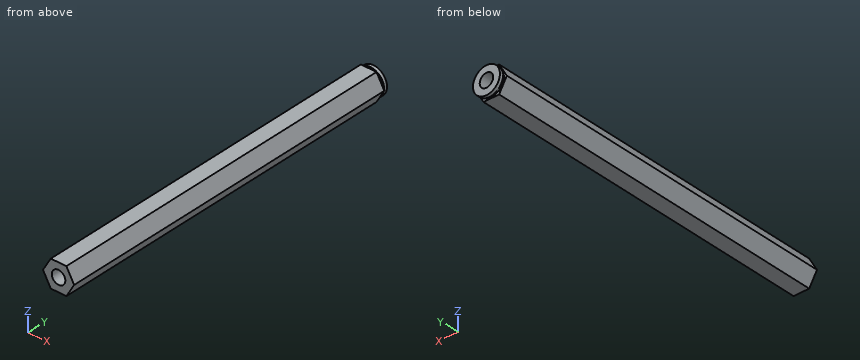
```python
from build123d import *

# Parameters (mm, degrees)
F0_R     = 3.175
F1_DEPTH = 168.275


with BuildPart() as f1:
    # F0 (on Front) → F1 (new body)
    with BuildSketch(Plane.XZ):
        Polygon((3.6661742094, 6.35), (-3.6661742094, 6.35), (-7.3323484187, 0), (-3.6661742094, -6.35), (3.6661742094, -6.35), (7.3323484187, 0), align=None)
        Circle(F0_R, mode=Mode.SUBTRACT)
    extrude(amount=F1_DEPTH)

    # F2 (on Top) → F3 (revolve, cut)
    with BuildSketch(Plane.XY):
        Polygon((-6.35, -1.5875), (-6.35, 0), (-7.3323484187, 0), (-7.3323484187, -2.5781), (-5.9436, -2.5781), (-5.9436, -1.5875), align=None)
    revolve(axis=Axis((0, -1.28905, 0), (0, -1, 0)), mode=Mode.SUBTRACT)


solid = f1.part
```
Input: part model. Units: mm. Frame: model coordinates. Give positions to 0.01 mm unless a question says otherwise; leave off trailing zeros. Order: outer loops, then holes, each group sorted by start corner. A loop starts at its lowest first (then second) coordinate and runs counter-clockwise, first axis right, second up.
1. Section C-C on z = 1.5. Return the cut outline in (x, y) (1 decimal).
Derived:
outline: (-6.5, -168.3) - (-2.8, -168.3) - (-2.8, 0) - (-6.2, 0) - (-6.2, -1.6) - (-5.8, -1.6) - (-5.8, -2.6) - (-6.5, -2.6) - close; (2.8, -168.3) - (6.5, -168.3) - (6.5, -2.6) - (5.8, -2.6) - (5.8, -1.6) - (6.2, -1.6) - (6.2, 0) - (2.8, 0) - close
2. Section B-B on y = -94. Return the cut outline in (x, z) (3 decimals).
Derived:
outline: (-7.332, 0) - (-3.666, -6.35) - (3.666, -6.35) - (7.332, 0) - (3.666, 6.35) - (-3.666, 6.35) - close; hole circle Ø6.35 at (0, 0)
3. Material intervals for L1, parallel to Z at x = 0, y = -75.5 (3 decimals); L2, parallel to X at y = -7, z = 1 (3 decimals); L3, parallel to X at y = -21.5, z = -1.5, sorted ascending.
Derived:
L1: z = -6.35 to -3.175, 3.175 to 6.35
L2: x = -6.755 to -3.013, 3.013 to 6.755
L3: x = -6.47 to -2.8, 2.8 to 6.47
4. Pin query (flat end, axial travel): pin 1 (6 mm diameter, centred on x = 1.5, z = 1, fed in from +Y); pin 2 (4 mm diameter, centred on y = -68, z = -4, fed in from +X); pin 3 (1 mm diameter, centred on y = -104, z = -5, fed in from +X); pin 4 (3 mm diameter, centred on y = -54.5, z = 2.5, fed in from +X) (3 decimals). Return the tip coordinate at first contact, or that it passes through.
Derived:
pin 1: stops at y = 0
pin 2: stops at x = 6.18
pin 3: stops at x = 4.73
pin 4: stops at x = 6.755
